Input: dimensioned drawing with shaded views. Units: mm. Origin: part minimum x, y, z. Round coordinates to 2 decimals unless told otherwise and drop trailing zeros. Order: outer loops, then holes, each group sorted by start corner. A loop starts at its lowest first (then second) coordinate and runs counter-clockwise, first axis right, second up. Notation, with made-up numbers: M 8.25,14 L 54.25,14 A4 cw 54.25,21 Z; hole C -3,-8 d4. An arc over 180 degrees is marked long. Use one line per item in the form item = value. Start each with the question number.
Q1. Section B-B (y = 40). Return the cut outline in (x, z), plus the area to 3 significant figures.
Q2. Section A-A (x = 15). Return the cut outline in (y, z).
Q3. Section C-C (z = 2.15). Return the cut outline in (x, y).
Q4. Section D-D (x = 11.5). Return the cut outline in (y, z).
Q5. Material intervals for probe 1 along Y at (x, z) = (15, 1.05); probe 2 along Y at (x, z) = (14.25, 1.05); probe 3 along X at (y, z) = (39.5, 2.55), sorted ascending.
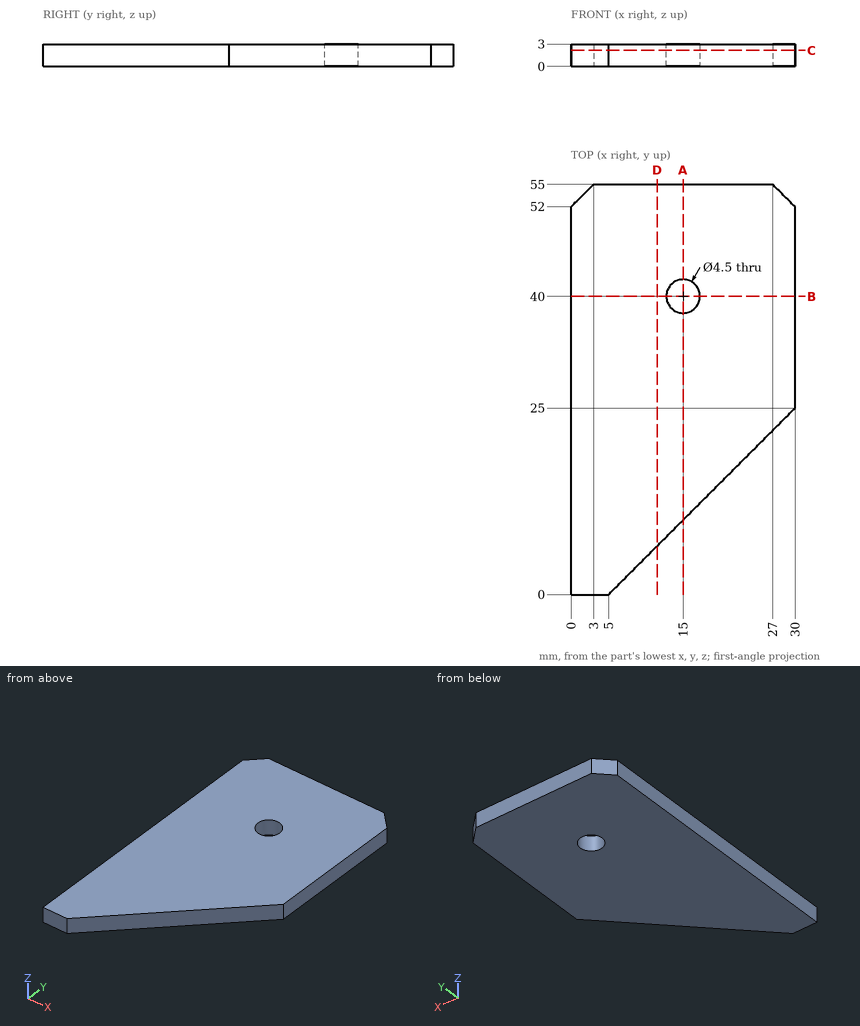
Results list:
q1.outline = M 0,0 L 12.75,0 L 12.75,3 L 0,3 Z; M 17.25,0 L 30,0 L 30,3 L 17.25,3 Z
q1.area = 76.5 mm2
q2.outline = M 10,0 L 37.75,0 L 37.75,3 L 10,3 Z; M 42.25,0 L 55,0 L 55,3 L 42.25,3 Z
q3.outline = M 0,0 L 5,0 L 30,25 L 30,52 L 27,55 L 3,55 L 0,52 Z; hole C 15,40 d4.5
q4.outline = M 6.5,0 L 55,0 L 55,3 L 6.5,3 Z
q5.probe_1 = 10 to 37.75, 42.25 to 55
q5.probe_2 = 9.25 to 37.88, 42.12 to 55
q5.probe_3 = 0 to 12.81, 17.19 to 30
